from build123d import *

# Parameters (mm, degrees)
SKETCH1_W           = 200
SKETCH1_H           = 150
BOSS_EXTRUDE1_DEPTH = 1
SKETCH2_R           = 1.5
SKETCH2_R_2         = 1.4
SKETCH2_W           = 14
SKETCH2_H           = 7
SKETCH2_W_2         = 12
SKETCH2_H_2         = 3
SKETCH2_W_3         = 23
SKETCH2_H_3         = 13.5
SKETCH2_W_4         = 2
SKETCH2_H_4         = 83
CUT_EXTRUDE1_DEPTH  = 1
SKETCH3_R           = 1.5
SKETCH3_W           = 5
SKETCH3_H           = 30
CUT_EXTRUDE2_DEPTH  = 10
SKETCH4_R           = 1.5
CUT_EXTRUDE3_DEPTH  = 10


with BuildPart() as part:
    # Sketch1 → Boss-Extrude1 (new body)
    with BuildSketch(Plane.XY):
        Rectangle(SKETCH1_W, SKETCH1_H)
    extrude(amount=BOSS_EXTRUDE1_DEPTH)

    # Sketch2 → Cut-Extrude1 (cut)
    with BuildSketch(Plane.XY.offset(1)):
        with Locations((-76.53, -67.5)):
            Circle(SKETCH2_R)
        with Locations((-59.53, -67.5)):
            Circle(SKETCH2_R)
        with Locations(Location((-59.53, 67.5, 0), (0, 0, 180))):
            Circle(SKETCH2_R)
        with Locations(Location((-76.53, 67.5, 0), (0, 0, 180))):
            Circle(SKETCH2_R)
        with Locations((-73, -40)):
            Circle(SKETCH2_R)
        with Locations((-63, -40)):
            Circle(SKETCH2_R)
        with Locations((-88.25346752, -58)):
            Circle(SKETCH2_R)
        with Locations((66.74653248, -58)):
            Circle(SKETCH2_R)
        with Locations(Location((66.74653248, 58, 0), (0, 0, 180))):
            Circle(SKETCH2_R)
        with Locations(Location((-88.25346752, 58, 0), (0, 0, 180))):
            Circle(SKETCH2_R)
        with Locations((64.8, 68.5)):
            Circle(SKETCH2_R_2)
        with Locations((92.2, 68.5)):
            Circle(SKETCH2_R_2)
        with Locations((85, 36.5)):
            Circle(SKETCH2_R)
        with Locations((85, -36.5)):
            Circle(SKETCH2_R)
        with Locations((-68, -55.5)):
            Rectangle(SKETCH2_W, SKETCH2_H)
        with Locations((-68, 55.5)):
            Rectangle(SKETCH2_W, SKETCH2_H)
        with Locations((-27, -13.75)):
            Rectangle(SKETCH2_W_2, SKETCH2_H_2)
        with Locations((-27, 13.75)):
            Rectangle(SKETCH2_W_2, SKETCH2_H_2)
        with Locations((78.5, 68.25)):
            Rectangle(SKETCH2_W_3, SKETCH2_H_3)
        with Locations((99, 0)):
            Rectangle(SKETCH2_W_4, SKETCH2_H_4)
    extrude(amount=-CUT_EXTRUDE1_DEPTH, mode=Mode.SUBTRACT)

    # Sketch3 → Cut-Extrude2 (cut)
    with BuildSketch(Plane.XY.offset(1)):
        with Locations((85.8, -69.04)):
            Circle(SKETCH3_R)
        with Locations((85.8, -59.04)):
            Circle(SKETCH3_R)
        with Locations((57.96, -62.5)):
            Circle(SKETCH3_R)
        with Locations((47.96, -62.5)):
            Circle(SKETCH3_R)
        with Locations((25.5, -0.49)):
            Rectangle(SKETCH3_W, SKETCH3_H)
    extrude(amount=-CUT_EXTRUDE2_DEPTH, mode=Mode.SUBTRACT)

    # Sketch4 → Cut-Extrude3 (cut)
    with BuildSketch(Plane.XY.offset(1)):
        with Locations((48, -12)):
            Circle(SKETCH4_R)
        with Locations((48, -56.04)):
            Circle(SKETCH4_R)
        with Locations((48, -32.04)):
            Circle(SKETCH4_R)
        with Locations((48, 12)):
            Circle(SKETCH4_R)
        with Locations((48, 31)):
            Circle(SKETCH4_R)
        with Locations((48, 55)):
            Circle(SKETCH4_R)
        with Locations((43, -25)):
            Circle(SKETCH4_R)
        with Locations((83, -25)):
            Circle(SKETCH4_R)
        with Locations((83, 25)):
            Circle(SKETCH4_R)
        with Locations((43, 25)):
            Circle(SKETCH4_R)
    extrude(amount=-CUT_EXTRUDE3_DEPTH, mode=Mode.SUBTRACT)


solid = part.part
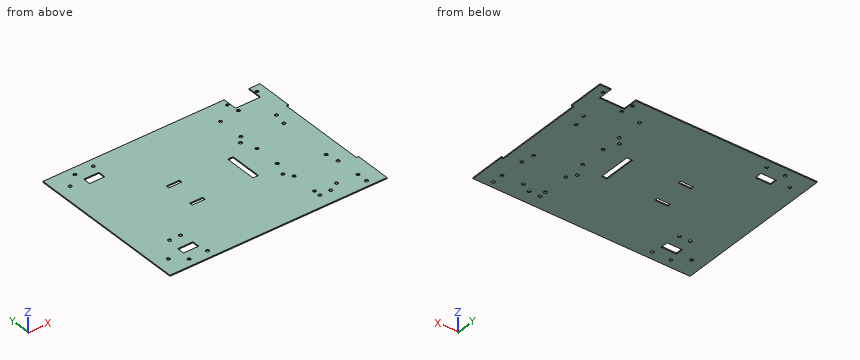
Read the model definition and answer for the solid it produces. Units are mm, in the model's axes. Round coordinates to 2 decimals unless told otherwise and drop trailing zeros. Write each loop counter-clockwise with the first axis right and the second up, starting at its lowest first coordinate (ties: lowest second). Pieces come first, ordered by that corner, then holes.
Q1. Straight lines are drawn through the part: line 1 (X direction, y = 58, z = 0.6); line 2 (Y direction, x = -29.5, z = 0.5); line 3 (X direction, y = -63, z = 0.6). For each, find the intervals that lie inside material, in ascending order.
Values:
line 1: x = -100 to -89.75, -86.75 to -75, -61 to 65.25, 68.25 to 100
line 2: y = -75 to -15.25, -12.25 to 12.25, 15.25 to 75
line 3: x = -100 to 46.55, 49.37 to 56.55, 59.37 to 100
Q2. Find section A-A on x = -67.5. Determine the outline of the cut face in (y, z).
Values:
outline: (-75, 0) - (-59, 0) - (-59, 1) - (-75, 1) - close; (-52, 0) - (52, 0) - (52, 1) - (-52, 1) - close; (59, 0) - (75, 0) - (75, 1) - (59, 1) - close
Q3. Find section B-B on z = 0.2. State how many separate pieces and enclosed holes the cut face has, and give its area (3 significant figures).
Values:
separate pieces: 1
enclosed holes: 33
area: 28,900 mm2
